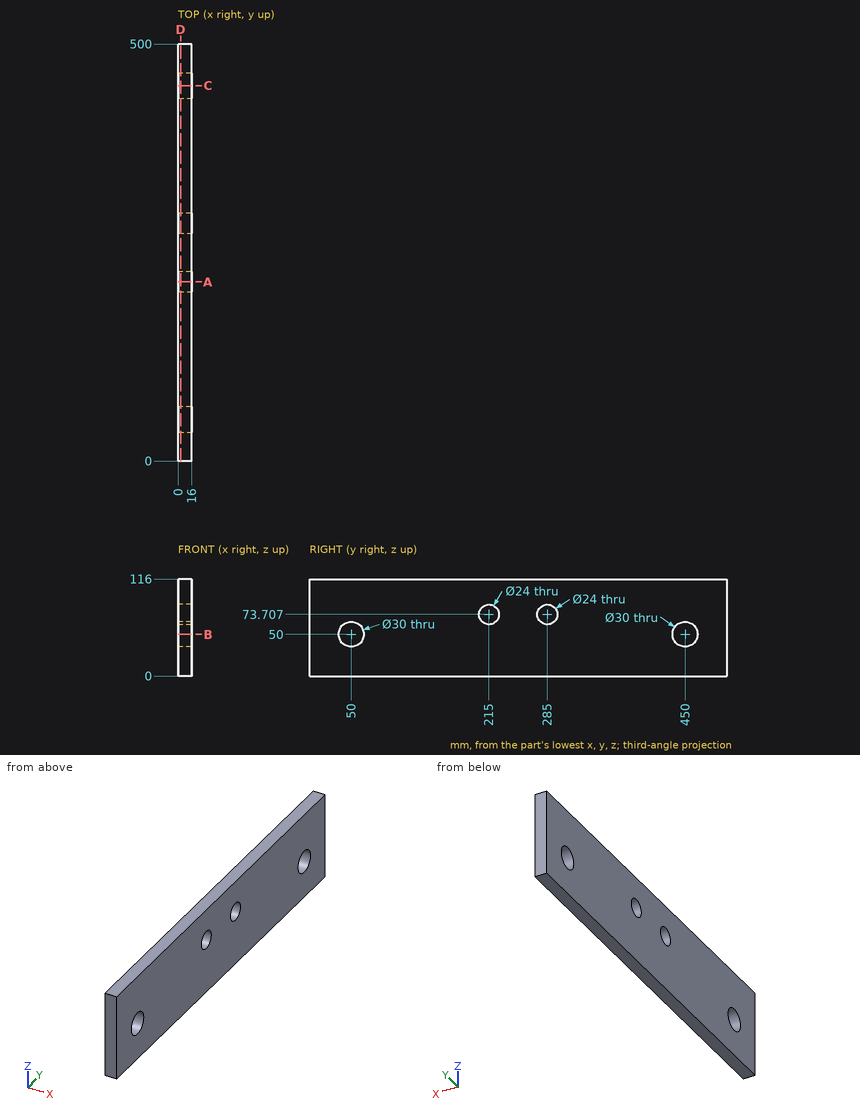
Verification items for this drawing (mm, ordinates from the low corner). Give positions to 0.01 mm unless a question says otherwise; leave off trailing zeros. Loops run counter-clockwise (first coordinate to the right, second up) from the corner with the lowest first, then second, coordinate; pieces in that order, holes last. Notation, with made-up numbers: M -21,38 L 1,38 A19 ccw 1,43 Z; hole C 67,-25 d10. An arc over 180 degrees is marked long. Write item = value, one per line.
(1) Sectioned sample at B-B, the plane z = 50. Record the cut outline in (x, y).
Answer below:
outline = M 0,0 L 16,0 L 16,35 L 0,35 Z; M 0,65 L 16,65 L 16,435 L 0,435 Z; M 0,465 L 16,465 L 16,500 L 0,500 Z
(2) Sectioned sample at C-C, the plane y = 450. Record the cut outline in (x, z).
Answer below:
outline = M 0,0 L 16,0 L 16,35 L 0,35 Z; M 0,65 L 16,65 L 16,116 L 0,116 Z
(3) Gauge pin test, flat end, axial feed: pin 1 Ø24 at (y, z) = (450, 50) entering from +X. Record the tip position at first contact, or that the pin passes through.
Answer below:
pin_1 = through
(4) Sectioned sample at D-D, the plane x = 3. Record the cut outline in (y, z), plus the area to 3 significant figures.
Answer below:
outline = M 0,0 L 500,0 L 500,116 L 0,116 Z; hole C 50,50 d30; hole C 215,73.71 d24; hole C 285,73.71 d24; hole C 450,50 d30
area = 55,700 mm2
(5) Material ranges on line 1 (Z direction, x = 4.75, y = 285); line 2 (Y direction, x = 10.5, z = 82) (1 decimal); line 3 (Y direction, x = 11, z = 39) (1 decimal), recorded low to high. Write a range as [from, to].
Answer below:
line_1 = [0, 61.71], [85.71, 116]
line_2 = [0, 206.3], [223.7, 276.3], [293.7, 500]
line_3 = [0, 39.8], [60.2, 439.8], [460.2, 500]
(6) Sectioned sample at A-A, the plane y = 215. Record the cut outline in (x, z).
Answer below:
outline = M 0,0 L 16,0 L 16,61.71 L 0,61.71 Z; M 0,85.71 L 16,85.71 L 16,116 L 0,116 Z
